from build123d import *

# Parameters (mm, degrees)
SKETCH_R        = 6
SKETCH_R_2      = 2.75
PAD_DEPTH       = 3.5
SKETCH003_R     = 9
SKETCH003_R_2   = 6
PAD001_DEPTH    = 6
FILLET_R        = 0.4
SKETCH004_R     = 2
POCKET_DEPTH    = 33.501
FILLET001_R     = 0.5
SKETCH005_W     = 1
SKETCH005_H     = 10
POCKET001_DEPTH = 13.001


with BuildPart() as part:
    # Sketch → Pad (new body, symmetric)
    with BuildSketch(Plane.XY):
        with BuildLine():
            Line((-2.5, 10), (2.5, 10))
            Line((19.468038, 5.300459), (2.5, 10))
            ThreePointArc((19.756482, -5.211983), (23.497931, 0.150854), (19.468038, 5.300459))
            Line((19.756482, -5.211983), (10, -8.5))
            Line((10, -14), (10, -8.5))
            Line((-10, -14), (10, -14))
            Line((-10, -14), (-10, -8.5))
            Line((-10, -8.5), (-19.756482, -5.211983))
            ThreePointArc((-19.468038, 5.300459), (-23.497931, 0.150854), (-19.756482, -5.211983))
            Line((-19.468038, 5.300459), (-2.5, 10))
        make_face()
        Circle(SKETCH_R, mode=Mode.SUBTRACT)
        with Locations((18, 0)):
            Circle(SKETCH_R_2, mode=Mode.SUBTRACT)
        with Locations((-18, 0)):
            Circle(SKETCH_R_2, mode=Mode.SUBTRACT)
    extrude(amount=PAD_DEPTH, both=True)

    # Sketch003 → Pad001 (join)
    with BuildSketch(Plane.XY.offset(3.5)):
        Circle(SKETCH003_R)
        Circle(SKETCH003_R_2, mode=Mode.SUBTRACT)
    extrude(amount=PAD001_DEPTH)

    # Fillet
    fillet_edges = [part.edges().sort_by_distance(p)[0] for p in [
        (10, -14, 0),
        (-10, -14, 0),
    ]]
    fillet(fillet_edges, radius=FILLET_R)

    # Sketch004 (on Face10 of Pad001) → Pocket (cut, through all)
    with BuildSketch(Plane.YZ.offset(10)):
        with Locations((-11.25, 0)):
            Circle(SKETCH004_R)
    extrude(amount=-POCKET_DEPTH, mode=Mode.SUBTRACT)

    # Fillet001
    fillet001_edges = [part.edges().sort_by_distance(p)[0] for p in [
        (-9, 0, 9.5),
        (-6, 0, 9.5),
    ]]
    fillet(fillet001_edges, radius=FILLET001_R)

    # Sketch005 (on Face3 of Fillet001) → Pocket001 (cut, through all)
    with BuildSketch(Plane(origin=(0, 0, -3.5), x_dir=(1, 0, 0), z_dir=(0, 0, -1))):
        with Locations((0, 10)):
            Rectangle(SKETCH005_W, SKETCH005_H)
    extrude(amount=-POCKET001_DEPTH, mode=Mode.SUBTRACT)


solid = part.part
Could you check a few things on this model? Use its own coordinates, in mm. A direction names the side the tool comes from. Give positions to 0.01 mm unless a question says otherwise; leave off trailing zeros. Order: outer loops, then holes, each group sorted by start corner. A loop starts at its lowest first (then second) coordinate and runs counter-clockwise, first axis right, second up. Notation, with made-up numbers: (-34, 29) -> (2, 29) arc R16 ccw to (2, 33) -> close; hole circle Ø4 at (73, 64). An arc over 180 degrees is marked (long way). Answer in a Markdown table with one row per item. Add a question column.
Item 1: Please list where these lines run through material, in increasing order: probe 1 along Z at (x, y) = (3.5, -11.25); probe 2 along X at (y, z) = (-2, -0.75); probe 3 along X at (y, z) = (-1, 3.25).
Item 2: Imagine slicing it at B-B (y = -11.25). List the corners of the cut face in (x, z) for me.
Item 3: Imagine slicing it at C-C (x = 18). List the corners of the cut face in (y, z) for me, and give its area (3 significant figures).
Item 4: Imagine slicing it at A-A (z = -1). List the corners of the cut face in (x, y) for me.
Item 5: We'd pull the mould along Z, two halves only. Please class faces 1 (the flat face through (0.5, -9, 1)), 2 (the cylindrical face through (5.316, -12.837, -1.217)), 3 (the flat face through (6, -7, 3.5)): pulls with the +Z half, pulls with the -Z half, needs draft (parallel to the pull), parting line crosses it, or undercut.
Item 6: Imagine slicing it at D-D (z = 2.5). List the corners of the cut face in (x, y) for me.
Item 7: For faces 4 (the flat face through (-10, -9, 1)), 5 (the flat face through (-0.5, -9, 1)), 6 (the cylindrical face through (0, 6, 3)), which set-ups out of +Z, -Z, +X, -X, +Y, -Y let a thin tool reach every point of the face, with its end or its side?
Item 8: I'm going to push flat-ended pins straight in: P1, Ø9, axis at x = 18, y = 0, coming from the +Z side; P2, Ø2.5, axis at y = -10, z = 0, coming from the +X side; P3, Ø2, axis at y = -10.5, z = 3.5, coming from the -X side; P4, Ø2.5, axis at y = -11.25, z = 0, coming from the -X side. Where does each tip first touch, or does it pass through?
Result:
| question | item | result |
|---|---|---|
| 1 | probe 1 | -3.5 to -2, 2 to 3.5 |
| 1 | probe 2 | -23.12 to -19.89, -16.11 to -5.66, 5.66 to 16.11, 19.89 to 23.12 |
| 1 | probe 3 | -23.41 to -20.56, -15.44 to -5.92, 5.92 to 15.44, 20.56 to 23.41 |
| 2 | outline | (-10, -3.5) -> (-0.5, -3.5) -> (-0.5, -2) -> (-10, -2) -> close; (-10, 2) -> (-0.5, 2) -> (-0.5, 3.5) -> (-10, 3.5) -> close; (0.5, -3.5) -> (10, -3.5) -> (10, -2) -> (0.5, -2) -> close; (0.5, 2) -> (10, 2) -> (10, 3.5) -> (0.5, 3.5) -> close |
| 3 | outline | (-5.8, -3.5) -> (-2.75, -3.5) -> (-2.75, 3.5) -> (-5.8, 3.5) -> close; (2.75, -3.5) -> (5.71, -3.5) -> (5.71, 3.5) -> (2.75, 3.5) -> close |
| 3 | area | 42.1 mm2 |
| 4 | outline | (-19.76, -5.21) -> (-10, -8.5) -> (-10, -9.52) -> (-0.5, -9.52) -> (-0.5, -5.98) arc R6 cw (long way) to (0.5, -5.98) -> (0.5, -9.52) -> (10, -9.52) -> (10, -8.5) -> (19.76, -5.21) arc R5.5 ccw to (19.47, 5.3) -> (2.5, 10) -> (-2.5, 10) -> (-19.47, 5.3) arc R5.5 ccw to start; (-10, -13.6) arc R0.4 ccw to (-9.6, -14) -> (-0.5, -14) -> (-0.5, -12.98) -> (-10, -12.98) -> close; (0.5, -14) -> (9.6, -14) arc R0.4 ccw to (10, -13.6) -> (10, -12.98) -> (0.5, -12.98) -> close; hole circle Ø5.5 at (-18, 0); hole circle Ø5.5 at (18, 0) |
| 5 | face 1 | needs draft |
| 5 | face 2 | undercut |
| 5 | face 3 | pulls with the +Z half |
| 6 | outline | (-19.76, -5.21) -> (-10, -8.5) -> (-10, -13.6) arc R0.4 ccw to (-9.6, -14) -> (-0.5, -14) -> (-0.5, -5.98) arc R6 cw (long way) to (0.5, -5.98) -> (0.5, -14) -> (9.6, -14) arc R0.4 ccw to (10, -13.6) -> (10, -8.5) -> (19.76, -5.21) arc R5.5 ccw to (19.47, 5.3) -> (2.5, 10) -> (-2.5, 10) -> (-19.47, 5.3) arc R5.5 ccw to start; hole circle Ø5.5 at (-18, 0); hole circle Ø5.5 at (18, 0) |
| 7 | face 4 | +Z, -Z, -X, -Y |
| 7 | face 5 | +Z, -Z, -Y |
| 7 | face 6 | +Z, -Z |
| 8 | P1 | z = 3.5 |
| 8 | P2 | x = 10 |
| 8 | P3 | x = -10 |
| 8 | P4 | through |
